The listing builds one solid part. Answer for the finished solid, in the listing's coordinates (mm). Coordinates: 2 decimals unless noted, no trailing zeros. Loops run counter-clockwise (first coordinate to the right, second up) from the corner with the lowest first, then second, coordinate; pieces in that order, holes last. Notation, with made-up numbers: (49.5, -30) - (92.5, -30) arc R30 ccw to (92.5, -6) - close; hole circle Ø8 at (0, 69.5). An arc over 180 degrees is marked (long way). Write each question's results on one line, items separated by ' | '. Start each with the question number.
(1) Find section A-A on x = 0. Determine the outline of the cut face in (y, z), then the cut area to 3 significant figures.
(2) Find section C-C on z = 11. Determine the outline of the cut face in (x, y).
(3) Given pin 1 Ø1.8 at (x, z) = (-9.53, 5.5) entering from -Y, flat-ended and moving along its own axis, determine where the tip first touches the part or whether it passes through.
(4) Consider line 1 (X direction, y = 0.3, z = 5.5); line 2 (X direction, y = 0.1, z = 5); line 3 (X direction, y = 0.55, z = 11). Determine where each line is inside the solid, lowest interval first. Write a range as from..to.
(5) Find section D-D on y = 0.65. Determine the outline of the cut face in (x, z), then the cut area to 3 significant figures.
(6) Determine the mould class of faces 1 (the cylindrical face through (-10.5, 0.49, 5.28)), 2 (the cylindrical face through (-0.279, 0.493, 12.697)), 3 (the flat face through (-10.1, 0.5, 0)) for opening direction X: released by +X, released by -X, zero draft, split by the parting line, or undercut.
(7) Find section B-B on z = 5.5. Determine the outline of the cut face in (x, y).
from build123d import *

# Parameters (mm, degrees)
SKETCH1_R               = 12.7
BOSS_EXTRUDE1_DEPTH     = 1
CUT_EXTRUDE1_DEPTH      = 18.98832955
CUT_EXTRUDE1_DEPTH_BACK = 18.98832955
SKETCH19_R              = 1
CUT_EXTRUDE2_DEPTH      = 18.98832955
CUT_EXTRUDE2_DEPTH_BACK = 18.98832955
SKETCH20_R              = 7.5
SKETCH21_W              = 65.874202484
SKETCH21_H              = 51.979273979
CUT_EXTRUDE3_DEPTH      = 18.98832955


with BuildPart() as part:
    # Sketch1 → Boss-Extrude1 (new body)
    with BuildSketch(Plane(origin=(0, 0, 0), x_dir=(1, 0, 0), z_dir=(0, 1, 0))):
        with Locations(Location((0, 0, 0), (0, 0, 270))):
            Circle(SKETCH1_R)
    extrude(amount=BOSS_EXTRUDE1_DEPTH)

    # Sketch19 → Cut-Extrude1 (cut, two sides: drawn at the far end of the back side and taken through both)
    with BuildSketch(Plane(origin=(0, 1, 0), x_dir=(1, 0, 0), z_dir=(0, 1, 0)).offset(-CUT_EXTRUDE1_DEPTH_BACK)):
        with Locations(Location((0, 11, 0), (0, 0, 270))):
            Circle(SKETCH19_R)
        with Locations(Location((9.526279442, 5.5, 0), (0, 0, 270))):
            Circle(SKETCH19_R)
        with Locations(Location((9.526279442, -5.5, 0), (0, 0, 270))):
            Circle(SKETCH19_R)
        with Locations(Location((0, -11, 0), (0, 0, 270))):
            Circle(SKETCH19_R)
        with Locations(Location((-9.526279442, -5.5, 0), (0, 0, 270))):
            Circle(SKETCH19_R)
        with Locations(Location((-9.526279442, 5.5, 0), (0, 0, 270))):
            Circle(SKETCH19_R)
    extrude(amount=CUT_EXTRUDE1_DEPTH + CUT_EXTRUDE1_DEPTH_BACK, mode=Mode.SUBTRACT)

    # Sketch20 → Cut-Extrude2 (cut, two sides: drawn at the far end of the back side and taken through both)
    with BuildSketch(Plane(origin=(0, 1, 0), x_dir=(1, 0, 0), z_dir=(0, 1, 0)).offset(-CUT_EXTRUDE2_DEPTH_BACK)):
        with Locations(Location((0, 0, 0), (0, 0, 270))):
            Circle(SKETCH20_R)
    extrude(amount=CUT_EXTRUDE2_DEPTH + CUT_EXTRUDE2_DEPTH_BACK, mode=Mode.SUBTRACT)

    # Sketch21 → Cut-Extrude3 (cut, through all)
    with BuildSketch(Plane.XY):
        with Locations((-3.816154381, 6.321647006)):
            Rectangle(SKETCH21_W, SKETCH21_H)
    extrude(amount=-CUT_EXTRUDE3_DEPTH, mode=Mode.SUBTRACT)


solid = part.part
Values:
1) outline: (0, 7.5) - (1, 7.5) - (1, 10) - (0, 10) - close; (0, 12) - (1, 12) - (1, 12.7) - (0, 12.7) - close | area: 3.20 mm²
2) outline: (-6.35, 0) - (-1, 0) - (-1, 1) - (-6.35, 1) - close; (1, 0) - (6.35, 0) - (6.35, 1) - (1, 1) - close
3) pin 1: passes through
4) line 1: x = -11.45..-10.53, -8.53..-5.1, 5.1..8.53, 10.53..11.45 | line 2: x = -11.67..-10.39, -8.66..-5.59, 5.59..8.66, 10.39..11.67 | line 3: x = -6.35..-1, 1..6.35
5) outline: (-12.7, 0) - (-7.5, 0) arc R7.5 cw to (7.5, 0) - (12.7, 0) arc R12.7 ccw to start; hole circle Ø2 at (-9.53, 5.5); hole circle Ø2 at (0, 11); hole circle Ø2 at (9.53, 5.5) | area: 156 mm²
6) face 1: undercut | face 2: split by the parting line | face 3: zero draft
7) outline: (-11.45, 0) - (-10.53, 0) - (-10.53, 1) - (-11.45, 1) - close; (-8.53, 0) - (-5.1, 0) - (-5.1, 1) - (-8.53, 1) - close; (5.1, 0) - (8.53, 0) - (8.53, 1) - (5.1, 1) - close; (10.53, 0) - (11.45, 0) - (11.45, 1) - (10.53, 1) - close
